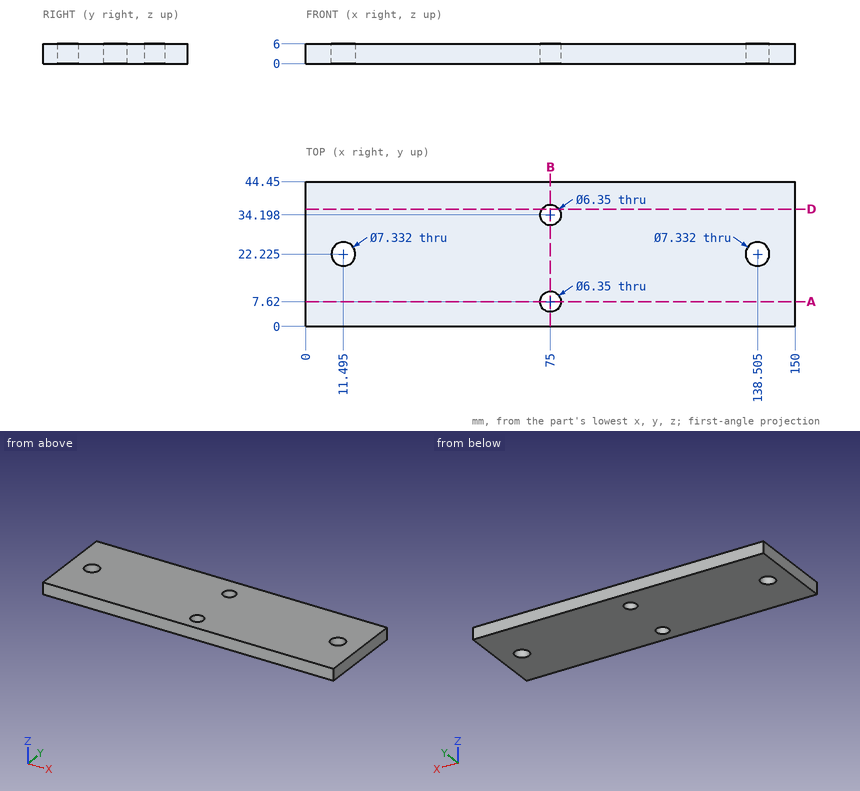
Drawing for the job (mm, zero at the part's lowest x, y, z). Give positions to 0.01 mm unless a question says otherwise; leave off trailing zeros. Loops run counter-clockwise (first coordinate to the right, second up) from the corner with the lowest first, then second, coordinate; pieces in that order, holes last. Notation, with made-up numbers: (85.25, 87) - (95.25, 87) arc R28 ccw to (95.25, 107) - close; hole circle Ø3 at (7.5, 49). An arc over 180 degrees is marked (long way). Write item = value, one per line. Start each with the question number.
1) Band-saw the part on D-D on y = 36. Give the cut face in (x, z).
2) Band-saw the part on B-B on x = 75. Count the separate pieces of the cut face and the enclosed holes in it.
3) Band-saw the part on A-A on y = 7.62. Give the cut face in (x, z) (1 decimal), plus the area to 3 significant figures.
4) Probe probe 1 along X at (y, z) = (20, 2.9); probe 2 along X at (y, z) = (23, 2.45); probe 3 along X at (y, z) = (7.5, 4.25). List the from-to ranges inside material, lowest first. Write a range as from..to.
Final values:
q1.outline = (0, 0) - (72.39, 0) - (72.39, 6) - (0, 6) - close; (77.61, 0) - (150, 0) - (150, 6) - (77.61, 6) - close
q2.separate_pieces = 3
q2.enclosed_holes = 0
q3.outline = (0, 0) - (71.8, 0) - (71.8, 6) - (0, 6) - close; (78.2, 0) - (150, 0) - (150, 6) - (78.2, 6) - close
q3.area = 862 mm²
q4.probe_1 = 0..8.58, 14.41..135.59, 141.42..150
q4.probe_2 = 0..7.91, 15.08..134.92, 142.09..150
q4.probe_3 = 0..71.83, 78.17..150
